Design review of the part shown in the three views and the two pictorial views. Dimensions are in mm from the part's minimum x, y and z. A direction names the side the tool comes from. Round coordinates to 2 decimals unless told otherwise and drop trailing zeros. Write each loop counter-clockwise with the first axis right and the second up, starting at its lowest first coordinate (ties: lowest second). Pieces come first, ordered by that corner, then holes. Notation, with made-up numbers: (57, -20.75) - (100, -20.75) arc R15 ccw to (100, -8.75) - close; hole circle Ø9 at (77.25, 85). An arc over 180 degrees is marked (long way). Use one line per item in the form item = value.
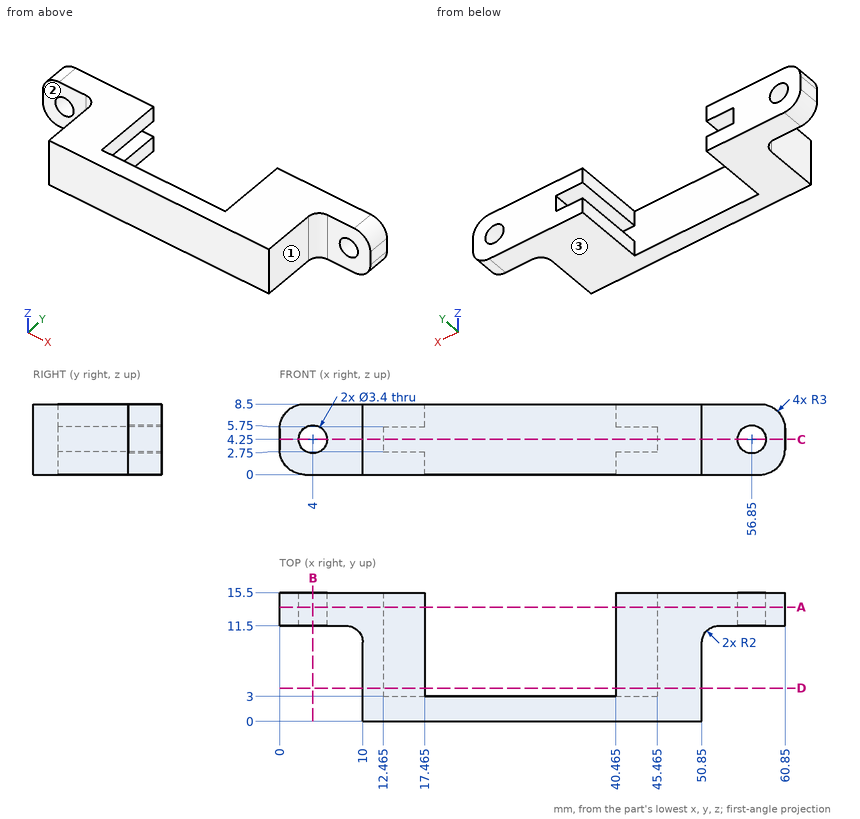
Q1. Machinability: for the marked faces 1, 2 and 3, which of the approach directions +Z, -Z, +X, -X, +Y, -Y give a long, thin tool a straight path to every point of the face, cutting with its end or side? Answer none if there is none.
Calculated:
face_1 = +Z, -Z, +X, -Y
face_2 = +Z, -Z, -X, -Y
face_3 = -Z, +X, -X, +Y, -Y
Q2. We need section C-C on z = 4.25. Write out the cut boundary in (x, y) (3 decimals), then the cut area to 3 significant figures.
Calculated:
outline = (0, 11.5) - (2.3, 11.5) - (2.3, 15.5) - (0, 15.5) - close; (5.7, 11.5) - (8, 11.5) arc R2 cw to (10, 9.5) - (10, 0) - (50.85, 0) - (50.85, 9.5) arc R2 cw to (52.85, 11.5) - (55.15, 11.5) - (55.15, 15.5) - (45.465, 15.5) - (45.465, 3) - (12.465, 3) - (12.465, 15.5) - (5.7, 15.5) - close; (58.55, 11.5) - (60.85, 11.5) - (60.85, 15.5) - (58.55, 15.5) - close
area = 275 mm2
Q3. For P1, Ø4, axis at y = 7, z = 6, coming from the +X side; P2, Ø2.5, axis at x = 56.5, z = 5, coming from the -Y side; P3, Ø0.8, axis at y = 11.5, z = 8, coming from the +X side, all flat-tipped, find the tip position at first contact; note any pin that passes through.
Calculated:
P1 = 50.85
P2 = 11.5
P3 = 59.99
Q4. We need section A-A on y = 13.75. Write out the cut boundary in (x, z) (3 decimals).
Calculated:
outline = (0, 3) arc R3 ccw to (3, 0) - (17.465, 0) - (17.465, 2.75) - (12.465, 2.75) - (12.465, 5.75) - (17.465, 5.75) - (17.465, 8.5) - (3, 8.5) arc R3 ccw to (0, 5.5) - close; (40.465, 0) - (57.85, 0) arc R3 ccw to (60.85, 3) - (60.85, 5.5) arc R3 ccw to (57.85, 8.5) - (40.465, 8.5) - (40.465, 5.75) - (45.465, 5.75) - (45.465, 2.75) - (40.465, 2.75) - close; hole circle Ø3.4 at (4, 4.25); hole circle Ø3.4 at (56.85, 4.25)
Q5. We need section D-D on y = 4. Write out the cut boundary in (x, z) (3 decimals), then the cut area to 3 significant figures.
Calculated:
outline = (10, 0) - (17.465, 0) - (17.465, 2.75) - (12.465, 2.75) - (12.465, 5.75) - (17.465, 5.75) - (17.465, 8.5) - (10, 8.5) - close; (40.465, 0) - (50.85, 0) - (50.85, 8.5) - (40.465, 8.5) - (40.465, 5.75) - (45.465, 5.75) - (45.465, 2.75) - (40.465, 2.75) - close
area = 122 mm2
Q6. To check wall thickness, follow line 1 along X through (y, z) = (14.05, 4.25) (3 decimals); line 2 along X through (y, z) = (8.25, 7.5) (3 decimals); line 3 along Z through (x, y) = (56.85, 12.9). State the ranges of each line that lie inside material, in increasing order. Write a range as from..to.
Calculated:
line_1 = 0..2.3, 5.7..12.465, 45.465..55.15, 58.55..60.85
line_2 = 10..17.465, 40.465..50.85
line_3 = 0..2.55, 5.95..8.5
Q7. We need section B-B on x = 4. Write out the cut boundary in (y, z).
Calculated:
outline = (11.5, 0) - (15.5, 0) - (15.5, 2.55) - (11.5, 2.55) - close; (11.5, 5.95) - (15.5, 5.95) - (15.5, 8.5) - (11.5, 8.5) - close
